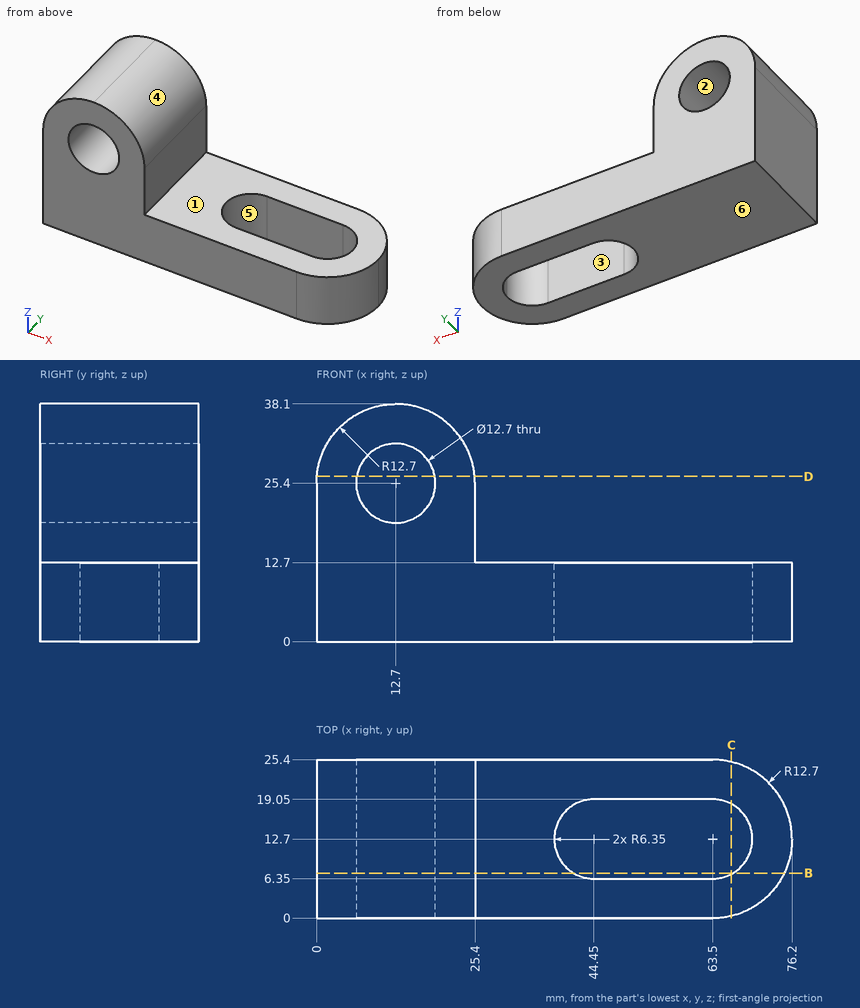
Design review of the part shown in the three views and the two pictorial views. Dimensions are in mm from the part's minimum x, y and z. A direction names the side the tool comes from. Round coordinates to 2 decimals unless told otherwise and drop trailing zeros. Loops run counter-clockwise (first coordinate to the right, second up) from the corner with the lowest first, then second, coordinate; pieces in that order, holes last. Notation, with made-up numbers: (34.25, 41.25) - (48.25, 41.25) arc R28 ccw to (48.25, 70.25) - close; hole circle Ø6 at (43.5, -23.5). An arc over 180 degrees is marked (long way). One line per item, written item: value. Start each with the question number.
Item 1: For L1, parallel to Z at x = 12.7, y = 9.5; L2, parallel to Z at x = 9, y = 4.75; L3, parallel to X at y = 17.25, z = 12.5, list the stretches that pass through material, from the lowest coordinate up.
Item 2: For the marked faces 1, 2 and 3, list the 3-axis set-ups (+Z, -Z, +X, -X, +Y, -Y) from which the entire face can be reached by the end or side of a thin tool; tool diameter is ignored.
Item 3: Take a section at B-B (y = 7.25). State how many separate pieces and enclosed holes the cut face has, plus the area to 3 significant figures.
Item 4: Take a section at C-C (x = 66.5). Give the boundary of the cut face in (y, z).
Item 5: The part is to be moulded in two halves that separate along X. For the marked faces 4, 5 and 6, say which applies: +X half, -X half, draft (parallel to the pull), parting line (faces both ways), or undercut.
Item 6: Clearance check with flat-ended pins moving along their axes: pin 1 Ø4 at (y, z) = (17.5, 22.5) entering from +X; pin 2 Ø6 at (x, y) = (57, 7) entering from +Z; pin 3 Ø1.5 at (y, z) = (9, 34) entering from -X. State where each tip first meets the part, or that it passes through.
Item 7: Take a section at D-D (z = 26.5). Give the boundary of the cut face in (x, y).
Answer below:
1. L1: z = 0 to 19.05, 31.75 to 38.1
1. L2: z = 0 to 20.24, 30.56 to 37.55
1. L3: x = 0 to 40.02, 67.93 to 75.36
2. face 1: +Z, +X, +Y, -Y
2. face 2: +Y, -Y
2. face 3: +Z, -Z
3. separate pieces: 2
3. enclosed holes: 1
3. area: 1,080 mm2
4. outline: (0.36, 0) - (7.1, 0) - (7.1, 12.7) - (0.36, 12.7) - close; (18.3, 0) - (25.04, 0) - (25.04, 12.7) - (18.3, 12.7) - close
5. face 4: +X half
5. face 5: undercut
5. face 6: draft
6. pin 1: stops at x = 25.4
6. pin 2: stops at z = 12.7
6. pin 3: stops at x = 2.72
7. outline: (0.05, 0) - (6.45, 0) - (6.45, 25.4) - (0.05, 25.4) - close; (18.95, 0) - (25.35, 0) - (25.35, 25.4) - (18.95, 25.4) - close
